Part model, mm, in its own coordinate system. A direction names the side the tool comes from. Round coordinates to 2 decimals unless told otherwise and drop trailing zeros. Loops run counter-clockwise (first coordinate to the right, second up) from the corner with the lowest first, then second, coordinate; pieces in that order, holes last.
Autodesk Fusion 360 part; units mm, degrees
sketch "Esboço1" plane through (0, 0, 0) normal (0, 0, 1) x (1, 0, 0)
  line L0 (-52, 78) -> (52, 78)
  line L1 (52, 78) -> (52, -78)
  line L2 (52, -78) -> (-52, -78)
  line L3 (-52, -78) -> (-52, 78)
  dimension "d1" = 104
  dimension "d2" = 156
  dimension "d3" = 52
  dimension "d4" = 78
extrude "Extrusão1" add sketch "Esboço1" along normal blind 0.8
sketch "Esboço2" plane through (0, 0, 0.8) normal (0, 0, 1) x (-1, 0, 0)
  line L0 (52, 78) -> (-52, 78)
  line L1 (-52, 78) -> (-52, -78)
  line L2 (-52, -78) -> (52, -78)
  line L3 (52, -78) -> (52, 78)
  line L4 (-52, -78) -> (-42, -78)
  line L5 (-42, -78) -> (-42, -65)
  line L6 (-42, -65) -> (-52, -65)
  line L7 (-52, -65) -> (-52, -78)
  line L8 (0, -1.75) -> (0, -22.5)
  line L9 (42, -65) -> (52, -65)
  line L10 (42, -78) -> (42, -65)
  line L11 (52, -65) -> (52, -78)
  line L12 (52, -78) -> (42, -78)
  line L13 (42, -65) -> (-42, -65)
  line L14 (-42, -65) -> (-42, -78)
  line L15 (-42, -78) -> (42, -78)
  line L16 (42, -78) -> (42, -65)
  point P0 (52, -78)
  dimension "d7" = 10
  dimension "d8" = 13
extrude "Extrusão2" cut sketch "Esboço2" against normal blind 2 contours L2 L5 L10 L13 L14 L15 L16
sketch "Esboço3" plane through (0, 0, 0.8) normal (0, 0, 1) x (-1, 0, 0)
  line L0 (42, -65) -> (42, -78)
  line L1 (42, -78) -> (52, -78)
  line L2 (52, -78) -> (52, 78)
  line L3 (52, 78) -> (-52, 78)
  line L4 (-52, 78) -> (-52, -78)
  line L5 (-52, -78) -> (-42, -78)
  line L6 (-42, -78) -> (-42, -65)
  line L7 (-42, -65) -> (42, -65)
  line L8 (-33.25, 78) -> (33.25, 78)
  line L9 (33.25, 78) -> (33.25, 75)
  line L10 (33.25, 75) -> (-33.25, 75)
  line L11 (-33.25, 75) -> (-33.25, 78)
  arc A0 (33.25, 78) -> (52, -57.0483) centre (528.9728, 78) ccw
  line L12 (52, -57.0483) -> (52, 78)
  line L13 (0, -1.75) -> (0, -22.5)
  arc A1 (-52, -57.0483) -> (-33.25, 78) centre (-528.9728, 78) ccw
  line L14 (-33.25, 78) -> (-33.25, 75)
  line L15 (-52, -57.0483) -> (-52, 78)
  arc A2 (42, -65) -> (-0.2595, -15.5) centre (-8.1203, -65) ccw
  arc A3 (0.2595, -15.5) -> (-42, -65) centre (8.1203, -65) ccw
  point P0 (-52, 78)
  point P1 (-42, -65)
  point P2 (-0.2595, -15.5)
  dimension "d11" = 66.5
  dimension "d12" = 3
  dimension "d13" = 18.75
  dimension "d14" = 62.5
extrude "Extrusão3" cut sketch "Esboço3" against normal blind 2 contours L7 A2 A3 | L2 L3 A0 L12 | L3 L4 A1 L15
sketch "Esboço4" plane through (0, 0, 0.8) normal (0, 0, 1) x (-1, 0, 0)
  arc A0 (0, -15.5419) -> (-42, -65) centre (8.1203, -65) ccw
  arc A1 (42, -65) -> (0, -15.5419) centre (-8.1203, -65) ccw
  line L0 (42, -65) -> (42, -78)
  line L1 (42, -78) -> (52, -78)
  line L2 (52, -78) -> (52, -57.0483)
  arc A2 (33.25, 78) -> (52, -57.0483) centre (528.9728, 78) ccw
  line L3 (33.25, 78) -> (-33.25, 78)
  arc A3 (-52, -57.0483) -> (-33.25, 78) centre (-528.9728, 78) ccw
  line L4 (-52, -57.0483) -> (-52, -78)
  line L5 (-52, -78) -> (-42, -78)
  line L6 (-42, -78) -> (-42, -65)
  line L7 (-33.25, 78) -> (33.25, 78)
  line L8 (33.25, 78) -> (33.25, 73)
  line L9 (33.25, 73) -> (-33.25, 73)
  line L10 (-33.25, 73) -> (-33.25, 78)
  line L11 (-33.25, 78) -> (-27.25, 78)
  line L12 (-27.25, 78) -> (-27.25, 69)
  line L13 (-27.25, 69) -> (-33.25, 69)
  line L14 (-33.25, 69) -> (-33.25, 78)
  line L15 (33.25, 78) -> (27.25, 78)
  line L16 (27.25, 78) -> (27.25, 69)
  line L17 (27.25, 69) -> (33.25, 69)
  line L18 (33.25, 69) -> (33.25, 78)
  line L19 (-6, 78) -> (6, 78)
  line L20 (6, 78) -> (6, 69)
  line L21 (6, 69) -> (-6, 69)
  line L22 (-6, 69) -> (-6, 78)
  dimension "d17" = 66.5
  dimension "d18" = 5
  dimension "d19" = 6
  dimension "d20" = 6
  dimension "d21" = 12
  dimension "d22" = 6
extrude "Extrusão4" add sketch "Esboço4" along normal blind 9 contours L3 L7 L9 L10 L11 L12 L14 | L3 L7 L8 L9 L15 L16 L18 | L3 L7 L9 L19 L20 L22
sketch "Esboço5" plane through (-27.25, 0, 0) normal (1, 0, 0) x (0, 1, 0)
  line L0 (-78, 0.8) -> (-73, 0.8)
  line L1 (-73, 0.8) -> (-73, 9.8)
  line L2 (-73, 9.8) -> (-78, 9.8)
  circle A0 centre (-75.5, 7.8) radius 1.95
  line L3 (-78, 9.8) -> (-78, 0.8)
  point P0 (-75.5, 7.8)
  dimension "d25" = 2
  dimension "d27" = 3.9
  dimension "d43" = 2.5
extrude "Extrusão5" add sketch "Esboço5" along normal blind 60.5 contours A0
sketch "Esboço6" plane through (0, 0, 0.8) normal (0, 0, 1) x (-1, 0, 0)
  line L0 (-27.25, 78) -> (-27.25, 73)
  line L1 (-27.25, 73) -> (-33.25, 73)
  line L2 (-33.25, 73) -> (-33.25, 78)
  arc A0 (-52, -57.0483) -> (-33.25, 78) centre (-528.9728, 78) ccw
  line L3 (-52, -57.0483) -> (-52, -78)
  line L4 (-52, -78) -> (-42, -78)
  line L5 (-42, -78) -> (-42, -65)
  arc A1 (0, -15.5419) -> (-42, -65) centre (8.1203, -65) ccw
  arc A2 (42, -65) -> (0, -15.5419) centre (-8.1203, -65) ccw
  line L6 (42, -65) -> (42, -78)
  line L7 (42, -78) -> (52, -78)
  line L8 (52, -78) -> (52, -57.0483)
  arc A3 (33.25, 78) -> (52, -57.0483) centre (528.9728, 78) ccw
  line L9 (33.25, 78) -> (33.25, 73)
  line L10 (33.25, 73) -> (27.25, 73)
  line L11 (27.25, 73) -> (27.25, 78)
  line L12 (27.25, 78) -> (6, 78)
  line L13 (6, 78) -> (6, 73)
  line L14 (6, 73) -> (-6, 73)
  line L15 (-6, 73) -> (-6, 78)
  line L16 (-6, 78) -> (-27.25, 78)
  circle A4 centre (-47, -74.75) radius 2.375
  line L17 (0, -1.75) -> (0, -22.5)
  circle A5 centre (47, -74.75) radius 2.375
  point P0 (-47, -74.75)
  point P1 (47, -74.75)
  point P2 (52, -57.0483)
  point P3 (52, -78)
  point P4 (42, -78)
  point P5 (42, -65)
  dimension "d30" = 5
  dimension "d31" = 3.25
  dimension "d32" = 4.75
extrude "Extrusão6" add sketch "Esboço6" along normal blind 8.5 contours A4 | A5
sketch "Esboço7" plane through (0, 0, 9.3) normal (0, 0, 1) x (-1, 0, 0)
  circle A0 centre (-47, -74.75) radius 2.375
  circle A1 centre (-47, -74.75) radius 0.75
  line L0 (0, -1.75) -> (0, -22.5)
  circle A2 centre (47, -74.75) radius 0.75
  point P0 (47, -74.75)
  dimension "d36" = 1.5
  dimension "d37" = 1.625
extrude "Extrusão7" cut sketch "Esboço7" against normal blind 6 contours A1 | A2
sketch "Esboço8" plane through (0, 0, 0.8) normal (0, 0, 1) x (-1, 0, 0)
  circle A0 centre (47, -74.75) radius 2.375
  circle A1 centre (-47, -74.75) radius 2.375
  line L0 (-27.25, 78) -> (-27.25, 73)
  line L1 (-27.25, 73) -> (-33.25, 73)
  line L2 (-33.25, 73) -> (-33.25, 78)
  arc A2 (-52, -57.0483) -> (-33.25, 78) centre (-528.9728, 78) ccw
  line L3 (-52, -57.0483) -> (-52, -78)
  line L4 (-52, -78) -> (-42, -78)
  line L5 (-42, -78) -> (-42, -65)
  arc A3 (0, -15.5419) -> (-42, -65) centre (8.1203, -65) ccw
  arc A4 (42, -65) -> (0, -15.5419) centre (-8.1203, -65) ccw
  line L6 (42, -65) -> (42, -78)
  line L7 (42, -78) -> (52, -78)
  line L8 (52, -78) -> (52, -57.0483)
  arc A5 (33.25, 78) -> (52, -57.0483) centre (528.9728, 78) ccw
  line L9 (33.25, 78) -> (33.25, 73)
  line L10 (33.25, 73) -> (27.25, 73)
  line L11 (27.25, 73) -> (27.25, 78)
  line L12 (27.25, 78) -> (6, 78)
  line L13 (6, 78) -> (6, 73)
  line L14 (6, 73) -> (-6, 73)
  line L15 (-6, 73) -> (-6, 78)
  line L16 (-6, 78) -> (-27.25, 78)
  ellipse E0 centre (35.6344, 29.437) end of major axis (30.9782, 64.1259) minor radius 18.4551
  line L17 (40.2907, -5.2519) -> (30.9782, 64.1259) construction
  line L18 (53.9255, 31.8922) -> (17.3434, 26.9818) construction
  line L19 (0, -1.75) -> (0, -22.5)
  ellipse E1 centre (-35.6344, 29.437) end of major axis (-30.9782, 64.1259) minor radius 18.4551
  dimension "d42" = 70
extrude "Extrusão8" cut sketch "Esboço8" against normal blind 10 contours A2 E1 | A5 E0 picked at (-41.7722, 30.588) picked at (29.5401, 29.38)
sketch "Esboço9" plane through (0, 0, 0.8) normal (0, 0, 1) x (-1, 0, 0)
  ellipse E0 centre (35.6344, 29.437) end of major axis (30.9782, 64.1259) minor radius 18.4551 (33.4436, 64.1453) -> (40.2907, -5.2519) ccw
  arc A0 (33.25, 78) -> (33.4436, 64.1453) centre (528.9728, 78) ccw
  line L0 (33.25, 78) -> (33.25, 73)
  line L1 (33.25, 73) -> (27.25, 73)
  line L2 (27.25, 73) -> (27.25, 78)
  line L3 (27.25, 78) -> (6, 78)
  line L4 (6, 78) -> (6, 73)
  line L5 (6, 73) -> (-6, 73)
  line L6 (-6, 73) -> (-6, 78)
  line L7 (-6, 78) -> (-27.25, 78)
  line L8 (-27.25, 78) -> (-27.25, 73)
  line L9 (-27.25, 73) -> (-33.25, 73)
  line L10 (-33.25, 73) -> (-33.25, 78)
  arc A1 (-33.4436, 64.1453) -> (-33.25, 78) centre (-528.9728, 78) ccw
  ellipse E1 centre (-35.6344, 29.437) end of major axis (-30.9782, 64.1259) minor radius 18.4551 (-40.2907, -5.2519) -> (-33.4436, 64.1453) ccw
  arc A2 (-52, -57.0483) -> (-40.2907, -5.2519) centre (-528.9728, 78) ccw
  line L11 (-52, -57.0483) -> (-52, -78)
  line L12 (-52, -78) -> (-42, -78)
  line L13 (-42, -78) -> (-42, -65)
  arc A3 (0, -15.5419) -> (-42, -65) centre (8.1203, -65) ccw
  arc A4 (42, -65) -> (0, -15.5419) centre (-8.1203, -65) ccw
  line L14 (42, -65) -> (42, -78)
  line L15 (42, -78) -> (52, -78)
  line L16 (52, -78) -> (52, -57.0483)
  arc A5 (40.2907, -5.2519) -> (52, -57.0483) centre (528.9728, 78) ccw
  circle A6 centre (-47, -74.75) radius 2.375
  circle A7 centre (47, -74.75) radius 2.375
  line L17 (49.5, -63) -> (44.5, -63)
  line L18 (44.5, -63) -> (44.5, -61)
  line L19 (44.5, -61) -> (49.5, -61)
  line L20 (49.5, -61) -> (49.5, -63)
  line L21 (44.5, -59) -> (49.5, -59)
  line L22 (49.5, -59) -> (49.5, -57)
  line L23 (49.5, -57) -> (44.5, -57)
  line L24 (44.5, -57) -> (44.5, -59)
  line L25 (2.5, 70) -> (-2.5, 70)
  line L26 (-2.5, 70) -> (-2.5, 68)
  line L27 (-2.5, 68) -> (2.5, 68)
  line L28 (2.5, 68) -> (2.5, 70)
  line L29 (2.5, 66) -> (-2.5, 66)
  line L30 (-2.5, 66) -> (-2.5, 64)
  line L31 (-2.5, 64) -> (2.5, 64)
  line L32 (2.5, 64) -> (2.5, 66)
  dimension "d44" = 5
  dimension "d45" = 2
  dimension "d46" = 2.5
  dimension "d47" = 2.5
  dimension "d48" = 15
  dimension "d49" = 2.5
  dimension "d50" = 2
  dimension "d51" = 2
  dimension "d52" = 5
  dimension "d53" = 5
  dimension "d54" = 2
  dimension "d55" = 12
  dimension "d56" = 3.5
  dimension "d57" = 3
  dimension "d58" = 5
  dimension "d59" = 2
  dimension "d60" = 2
extrude "Extrusão9" cut sketch "Esboço9" against normal blind 0.4 contours L17 L18 L19 L20 | L21 L22 L23 L24 | L25 L26 L27 L28 | L29 L30 L31 L32
sketch "Esboço10" plane through (0, 61, 0) normal (0, 1, 0) x (-1, 0, 0)
  line L0 (49.5, 0.8) -> (44.5, 0.8)
  line L1 (44.5, 0.8) -> (44.5, 0.4)
  line L2 (44.5, 0.4) -> (49.5, 0.4)
  line L3 (49.5, 0.4) -> (49.5, 0.8)
  line L4 (44.5, 0.4) -> (49.5, 0.4)
  line L5 (49.5, 0.4) -> (49.5, 0.6)
  line L6 (49.5, 0.6) -> (44.5, 0.6)
  line L7 (44.5, 0.6) -> (44.5, 0.4)
  dimension "d63" = 5
extrude "Extrusão10" cut sketch "Esboço10" against normal blind 2 contours L1 L2 L3 L4 L5 L6 L7
sketch "Esboço11" plane through (0, -73, 0) normal (0, 1, 0) x (-1, 0, 0)
  line L0 (-6, 0.8) -> (6, 0.8)
  line L1 (6, 0.8) -> (6, 9.8)
  line L2 (6, 9.8) -> (-6, 9.8)
  line L3 (-6, 9.8) -> (-6, 0.8)
  line L4 (-2.5, 1.5) -> (2.5, 1.5)
  line L5 (2.5, 1.5) -> (2.5, 2.5)
  line L6 (2.5, 2.5) -> (-2.5, 2.5)
  line L7 (-2.5, 2.5) -> (-2.5, 1.5)
  dimension "d66" = 1
  dimension "d67" = 5
  dimension "d68" = 3.5
extrude "Extrusão11" cut sketch "Esboço11" against normal blind 20 contours L4 L5 L6 L7
sketch "Esboço12" plane through (0, -66, 0) normal (0, 1, 0) x (-1, 0, 0)
  line L0 (2.5, 0.8) -> (-2.5, 0.8)
  line L1 (-2.5, 0.8) -> (-2.5, 0.4)
  line L2 (-2.5, 0.4) -> (2.5, 0.4)
  line L3 (2.5, 0.4) -> (2.5, 0.8)
  line L4 (-2.5, 0.4) -> (2.5, 0.4)
  line L5 (2.5, 0.4) -> (2.5, 0.6)
  line L6 (2.5, 0.6) -> (-2.5, 0.6)
  line L7 (-2.5, 0.6) -> (-2.5, 0.4)
  dimension "d71" = 5
extrude "Extrusão12" cut sketch "Esboço12" against normal blind 2 contours L1 L2 L3 L4 L5 L6 L7
equation "d2 = 148 mm + 8 mm"
equation "d3 = ( 104 / 2 ) * 1 mm"
equation "d4 = ( ( 148 + 8 ) / 2 ) * 1 mm"
equation "d13 = ( ( 104 - 66.5 ) / 2 ) * 1 mm"
equation "d22 = ( 12 / 2 ) * 1 mm"
equation "d28 = 66.5 mm - 6 mm"
1) Wall check: line 1 along X through (y, z) = (74.75, 4.5) (3 decimals); line 2 along Z through (x, y) = (-11, -19.5); line 3 along Y through (x, z) = (47, 5) (3 decimals). Give the ranges that are in metal, low to high.
Values:
line 1: x = -49.375 to -47.75, -46.25 to -44.625, 44.625 to 46.25, 47.75 to 49.375
line 2: z = 0 to 0.8
line 3: y = 72.375 to 74, 75.5 to 77.125
2) Slice it at A-A, the plane z = 7.8. Give the cut face in (x, y) (3 decimals).
Values:
outline: circle Ø4.75 at (-47, 74.75); (-33.25, -78) - (-27.25, -78) - (-27.25, -77.45) - (-6, -77.45) - (-6, -78) - (6, -78) - (6, -77.45) - (27.25, -77.45) - (27.25, -78) - (33.25, -78) - (33.25, -73) - (27.25, -73) - (27.25, -73.55) - (6, -73.55) - (6, -73) - (-6, -73) - (-6, -73.55) - (-27.25, -73.55) - (-27.25, -73) - (-33.25, -73) - close; circle Ø4.75 at (47, 74.75); hole circle Ø1.5 at (-47, 74.75); hole circle Ø1.5 at (47, 74.75)
3) Mould opens along X. For faces 1 (the face through (-46, 74, 9.3)), 2 (the face through (-45.37, 30.94, 0.41)), 3 (the face through (-16.774, -77.047, 8.987)) say: released by +X, released by -X, zero draft, split by the parting line, or undercut.
Values:
face 1: zero draft
face 2: released by -X
face 3: undercut
4) Tool access for faces 4 (the face through (29.76, 32.18, 0.41)), 5 (the face through (0, -75, 1.5)), 6 (the face through (30, -73, 5)): list every direction of +Z, -Z, +X, -X, +Y, -Y with a clear straight run to the whole face (end or side of a thin tool).
Values:
face 4: +Z, -Z, +Y
face 5: +Y, -Y
face 6: +Z, +X, -X, +Y
5) Slice it at D-D, the plane y = -75.5. Give the number of separate pieces and of enclosed holes in the cut face, then the cut area to 3 significant figures.
Values:
separate pieces: 1
enclosed holes: 3
area: 430 mm2
6) Slice it at B-B, the plane y = 17.5. Give the cut face in (x, z), then the cut area to 3 significant figures.
Values:
outline: (-42.54, 0) - (-7.87, 0) - (-7.87, 0.8) - (-42.54, 0.8) - close; (7.87, 0) - (42.54, 0) - (42.54, 0.8) - (7.87, 0.8) - close
area: 55.5 mm2
7) Slice it at C-C, the plane x = 12.5. Give the cut face in (y, z).
Values:
outline: (-78, 0) - (19.32, 0) - (19.32, 0.8) - (-78, 0.8) - close; circle Ø3.9 at (-75.5, 7.8)
8) Drop flat-ended pins along their axis: pin 1 Ø3 at (x, y) = (26, 5.5) entering from +Z; pin 2 Ø5.5 at (y, z) = (-76, 5) entering from -X; pin 3 Ø5 at (x, z) = (29.5, 7) entering from +Y; pin 4 Ø1 at (x, z) = (34.5, 6) entering from -Y. Give the stop position or say it passes through.
Values:
pin 1: stops at z = 0.8
pin 2: stops at x = -33.25
pin 3: stops at y = -73
pin 4: passes through
